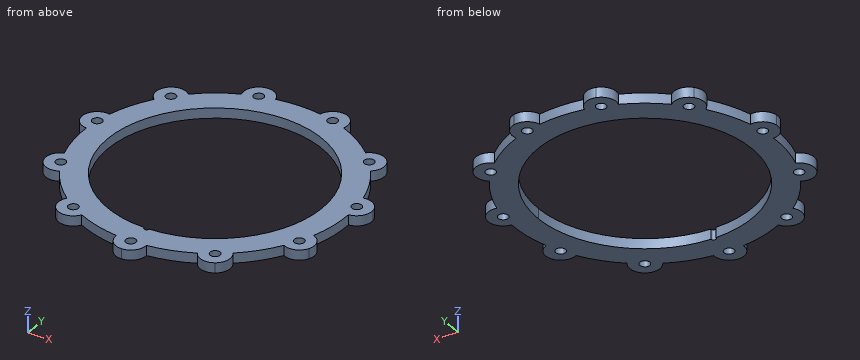
from build123d import *

# Parameters (mm, degrees)
SKETCH_1_R          = 42.7
SKETCH_1_R_2        = 2
EXTRUDE_1_DEPTH     = 4
SKETCH_2_R          = 1
CUT_EXTRUDE_1_DEPTH = 4


with BuildPart() as part:
    # 草图1 → 凸台-拉伸1 (new body)
    with BuildSketch(Plane.XY):
        with BuildLine():
            ThreePointArc((-57.90455435, 8.325418039), (-56.664135325, 3.740040393), (-52.478752132, 1.493510837))
            ThreePointArc((-52.478752132, 1.493510837), (-51.965625699, -7.471529009), (-49.932223308, -16.217986173))
            ThreePointArc((-49.932223308, -16.217986173), (-53.315148558, -19.552674205), (-53.213471728, -24.301778261))
            ThreePointArc((-53.213471728, -24.301778261), (-49.690922522, -27.488622249), (-44.95538855, -27.115734184))
            ThreePointArc((-44.95538855, -27.115734184), (-39.676852654, -34.380188532), (-33.237553958, -40.63883619))
            ThreePointArc((-33.237553958, -40.63883619), (-34.280583312, -45.27310175), (-31.627487821, -49.213331671))
            ThreePointArc((-31.627487821, -49.213331671), (-26.941192918, -49.989841552), (-23.159006743, -47.115925192))
            ThreePointArc((-23.159006743, -47.115925192), (-14.790959234, -50.373381115), (-5.990196072, -52.157142857))
            ThreePointArc((-5.990196072, -52.157142857), (-4.36217508, -56.619639374), (0, -58.5))
            ThreePointArc((0, -58.5), (4.36217508, -56.619639374), (5.990196072, -52.157142857))
            ThreePointArc((5.990196072, -52.157142857), (14.790959234, -50.373381115), (23.159006743, -47.115925192))
            ThreePointArc((23.159006743, -47.115925192), (26.941192918, -49.989841552), (31.627487821, -49.213331671))
            ThreePointArc((31.627487821, -49.213331671), (34.280583312, -45.27310175), (33.237553958, -40.63883619))
            ThreePointArc((33.237553958, -40.63883619), (39.676852654, -34.380188532), (44.95538855, -27.115734184))
            ThreePointArc((44.95538855, -27.115734184), (49.690922522, -27.488622249), (53.213471728, -24.301778261))
            ThreePointArc((53.213471728, -24.301778261), (53.315148558, -19.552674205), (49.932223308, -16.217986173))
            ThreePointArc((49.932223308, -16.217986173), (51.965625699, -7.471529009), (52.478752132, 1.493510837))
            ThreePointArc((52.478752132, 1.493510837), (56.664135325, 3.740040393), (57.90455435, 8.325418039))
            ThreePointArc((57.90455435, 8.325418039), (55.422530843, 12.375589248), (50.773764562, 13.351959864))
            ThreePointArc((50.773764562, 13.351959864), (47.755679756, 21.809288183), (43.34048271, 29.62857672))
            ThreePointArc((43.34048271, 29.62857672), (45.646885531, 33.781266636), (44.2113501, 38.309352936))
            ThreePointArc((44.2113501, 38.309352936), (39.933651182, 40.374690556), (35.494994318, 38.682752984))
            ThreePointArc((35.494994318, 38.682752984), (28.383642916, 44.165810474), (20.441916256, 48.35677884))
            ThreePointArc((20.441916256, 48.35677884), (20.137072107, 53.097179409), (16.481354575, 56.130338956))
            ThreePointArc((16.481354575, 56.130338956), (11.766119429, 55.555112887), (8.946814173, 51.732045351))
            ThreePointArc((8.946814173, 51.732045351), (0, 52.5), (-8.946814173, 51.732045351))
            ThreePointArc((-8.946814173, 51.732045351), (-11.766119429, 55.555112887), (-16.481354575, 56.130338956))
            ThreePointArc((-16.481354575, 56.130338956), (-20.137072107, 53.097179409), (-20.441916256, 48.35677884))
            ThreePointArc((-20.441916256, 48.35677884), (-28.383642916, 44.165810474), (-35.494994318, 38.682752984))
            ThreePointArc((-35.494994318, 38.682752984), (-39.933651182, 40.374690556), (-44.2113501, 38.309352936))
            ThreePointArc((-44.2113501, 38.309352936), (-45.646885531, 33.781266636), (-43.34048271, 29.62857672))
            ThreePointArc((-43.34048271, 29.62857672), (-47.755679756, 21.809288183), (-50.773764562, 13.351959864))
            ThreePointArc((-50.773764562, 13.351959864), (-55.422530843, 12.375589248), (-57.90455435, 8.325418039))
        make_face()
        Circle(SKETCH_1_R, mode=Mode.SUBTRACT)
        with Locations((-51.965625699, 7.471529009)):
            Circle(SKETCH_1_R_2, mode=Mode.SUBTRACT)
        with Locations((-39.676852654, 34.380188532)):
            Circle(SKETCH_1_R_2, mode=Mode.SUBTRACT)
        with Locations((-14.790959234, 50.373381115)):
            Circle(SKETCH_1_R_2, mode=Mode.SUBTRACT)
        with Locations((14.790959234, 50.373381115)):
            Circle(SKETCH_1_R_2, mode=Mode.SUBTRACT)
        with Locations((39.676852654, 34.380188532)):
            Circle(SKETCH_1_R_2, mode=Mode.SUBTRACT)
        with Locations((51.965625699, 7.471529009)):
            Circle(SKETCH_1_R_2, mode=Mode.SUBTRACT)
        with Locations((47.755679756, -21.809288183)):
            Circle(SKETCH_1_R_2, mode=Mode.SUBTRACT)
        with Locations((28.383642916, -44.165810474)):
            Circle(SKETCH_1_R_2, mode=Mode.SUBTRACT)
        with Locations((0, -52.5)):
            Circle(SKETCH_1_R_2, mode=Mode.SUBTRACT)
        with Locations((-28.383642916, -44.165810474)):
            Circle(SKETCH_1_R_2, mode=Mode.SUBTRACT)
        with Locations((-47.755679756, -21.809288183)):
            Circle(SKETCH_1_R_2, mode=Mode.SUBTRACT)
    extrude(amount=EXTRUDE_1_DEPTH)

    # 草图2 → 切除-拉伸1 (cut)
    with BuildSketch(Plane.XY.offset(4)):
        with Locations((0, -42.7)):
            Circle(SKETCH_2_R)
    extrude(amount=-CUT_EXTRUDE_1_DEPTH, mode=Mode.SUBTRACT)


solid = part.part
Geometry check sheet. Reference: the model listing, model coordinates, mm. Give positions to 0.01 mm unless a question says otherwise; leave off trailing zeros. Loops run counter-clockwise (first coordinate to the right, second up) from the corner with the lowest first, then second, coordinate; pieces in that order, holes last. Notation, with made-up numbers: (-26, -32.5) -> (31, -32.5) arc R4 cw to (31, -28.5) -> close; hole circle Ø7 at (64.25, 64.25). An arc over 180 degrees is marked (long way). Answer in a Markdown table with one row per item. Add a question column.
1) Cross-section at D-D on y = 46. Record the boundary of the cut face in (x, z), and give its area (3 significant figures).
2) Gauge pin test, flat ends, axial feed: P1, Ø6.5, axis at x = 14.79, y = 50.37, coming from the -Z side; P2, Ø1, axis at y = 16.5, z = 3.5, coming from the +X side; P3, Ø1.5, axis at y = 18.5, z = 1, coming from the -X side. Record the tip position at first contact, or that the pin passes through.
3) Material ranges on probe 1 along Y at (x, z) = (0, 2.9); probe 2 along X at (y, z) = (37.5, 2.1); probe 3 along Y at (x, z) = (46.5, 1.4), recorded low to high. Write a range as from..to.
4) Cross-section at A-A on y = -13. Record the boundary of the cut face in (x, z), and give its area (3 significant figures).
5) Cross-section at C-C on z = 1.65. State how many separate pieces and enclosed holes the cut face has, and give its area (3 significant figures).
6) Cross-section at B-B on x = -18.5. Record the boundary of the cut face in (y, z).
Outcome:
| question | item | result |
|---|---|---|
| 1 | outline | (-25.3, 0) -> (25.3, 0) -> (25.3, 4) -> (-25.3, 4) -> close |
| 1 | area | 202 mm^2 |
| 2 | P1 | stops at z = 0 |
| 2 | P2 | stops at x = 50 |
| 2 | P3 | stops at x = -49.41 |
| 3 | probe 1 | y = -58.5..-54.5, -50.5..-43.7, 42.7..52.5 |
| 3 | probe 2 | x = -44.8..-20.42, 20.42..44.8 |
| 3 | probe 3 | y = -27.68..-23.37, -20.25..24.37 |
| 4 | outline | (-50.87, 0) -> (-40.67, 0) -> (-40.67, 4) -> (-50.87, 4) -> close; (40.67, 0) -> (50.87, 0) -> (50.87, 4) -> (40.67, 4) -> close |
| 4 | area | 81.5 mm^2 |
| 5 | separate pieces | 1 |
| 5 | enclosed holes | 12 |
| 5 | area | 3,430 mm^2 |
| 6 | outline | (-49.13, 0) -> (-38.48, 0) -> (-38.48, 4) -> (-49.13, 4) -> close; (38.48, 0) -> (55.09, 0) -> (55.09, 4) -> (38.48, 4) -> close |
